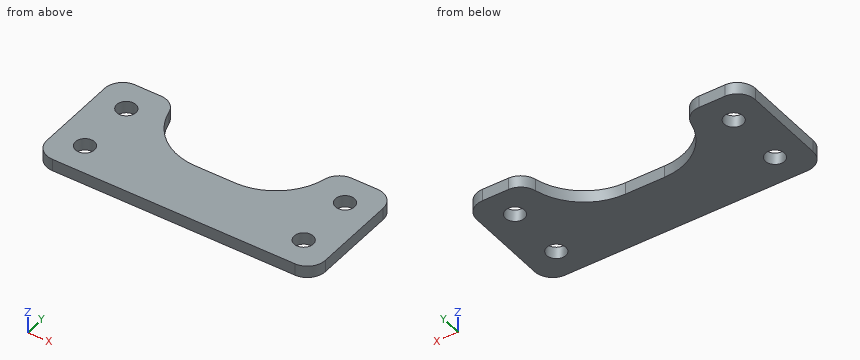
from build123d import *

# Parameters (mm, degrees)
SKETCH_1_R      = 1.6
EXTRUDE_1_DEPTH = 2
FILLET_1_R      = 10
FILLET_2_R      = 3


with BuildPart() as part:
    # ｽｹｯﾁ1 → ﾎﾞｽ - 押し出し1 (new body)
    with BuildSketch(Plane.XY):
        Polygon((0, 20), (0, 0), (46.6, 0), (46.6, 20), (36.6, 20), (36.6, 10), (10, 10), (10, 20), align=None)
        with Locations((5, 5)):
            Circle(SKETCH_1_R, mode=Mode.SUBTRACT)
        with Locations((41.6, 5)):
            Circle(SKETCH_1_R, mode=Mode.SUBTRACT)
        with Locations((5, 15)):
            Circle(SKETCH_1_R, mode=Mode.SUBTRACT)
        with Locations((41.6, 15)):
            Circle(SKETCH_1_R, mode=Mode.SUBTRACT)
    extrude(amount=EXTRUDE_1_DEPTH)

    # ﾌｨﾚｯﾄ1
    fillet_1_edges = [part.edges().sort_by_distance(p)[0] for p in [
        (36.6, 10, 1),
        (10, 10, 1),
    ]]
    fillet(fillet_1_edges, radius=FILLET_1_R - 0.0001)  # a hair under: the kernel refuses the full size

    # ﾌｨﾚｯﾄ2
    fillet_2_edges = [part.edges().sort_by_distance(p)[0] for p in [
        (46.6, 20, 1),
        (46.6, 0, 1),
        (0, 0, 1),
        (0, 20, 1),
        (10, 20, 1),
        (36.6, 20, 1),
    ]]
    fillet(fillet_2_edges, radius=FILLET_2_R)


solid = part.part
Can you work these out from the model? Positions are in its coordinate system, mm. Coordinates: 2 decimals unless noted, no trailing zeros. Write each loop counter-clockwise with the first axis right and the second up, starting at its lowest first coordinate (ties: lowest second). Pieces come first, ordered by that corner, then holes. Notation, with made-up numbers: (-24.5, 84.5) -> (31.5, 84.5) arc R13 ccw to (31.5, 109.5) -> close; hole circle Ø5 at (75, 57.25). An arc over 180 degrees is marked (long way). Answer as CSV lines item,"result".
1) If I drill on line 1 (Y direction, x = 41.6, z = 1); line 2 (X direction, y = 16.25, z = 1.5); line 3 (Y direction, x = 32, z = 1.4), over which ranges is the centre line in solid material (lowest first)? Write a range as from..to.
Check result:
line 1,"0..3.4, 6.6..13.4, 16.6..20"
line 2,"0..4, 6..10.73, 35.87..40.6, 42.6..46.6"
line 3,"0..11.58"
2) If we section it at A-A on y = 5: Please give me the cut outline in (x, z).
Check result:
outline,"(0, 0) -> (3.4, 0) -> (3.4, 2) -> (0, 2) -> close; (6.6, 0) -> (40, 0) -> (40, 2) -> (6.6, 2) -> close; (43.2, 0) -> (46.6, 0) -> (46.6, 2) -> (43.2, 2) -> close"
3) If we section it at B-B on x = 5: Please give me the cut outline in (y, z), then the cut area to 3 significant figures.
Check result:
outline,"(0, 0) -> (3.4, 0) -> (3.4, 2) -> (0, 2) -> close; (6.6, 0) -> (13.4, 0) -> (13.4, 2) -> (6.6, 2) -> close; (16.6, 0) -> (20, 0) -> (20, 2) -> (16.6, 2) -> close"
area,"27.2 mm²"
4) If we section it at C-C on y = 11.75: Please give me the cut outline in (x, z), then the cut area to 3 significant figures.
Check result:
outline,"(0, 0) -> (14.35, 0) -> (14.35, 2) -> (0, 2) -> close; (32.25, 0) -> (46.6, 0) -> (46.6, 2) -> (32.25, 2) -> close"
area,"57.4 mm²"
5) If we section it at D-D on y = 15: Please give me the cut outline in (x, z), then the cut area to 3 significant figures.
Check result:
outline,"(0, 0) -> (3.4, 0) -> (3.4, 2) -> (0, 2) -> close; (6.6, 0) -> (11.34, 0) -> (11.34, 2) -> (6.6, 2) -> close; (35.26, 0) -> (40, 0) -> (40, 2) -> (35.26, 2) -> close; (43.2, 0) -> (46.6, 0) -> (46.6, 2) -> (43.2, 2) -> close"
area,"32.6 mm²"
6) Will these pins go through, and if not, where does the flat tip stop? P1, Ø0.6, axis at x = 21.5, z = 1.5, coming from the +Y side; P2, Ø4, axis at x = 30, y = 10, coming from the -Z side; P3, Ø2.5, axis at x = 41.6, y = 15, coming from the +Z side.
Check result:
P1,"y = 10"
P2,"z = 0"
P3,"through"
